```python
from build123d import *

# Parameters (mm, degrees)
F0_W     = 102.9875054955
F0_H     = 41.0375036299
F1_DEPTH = 3
F2_W     = 102.9875054955
F2_H     = 41.0375036299
F3_DEPTH = 2


with BuildPart() as f1:
    # F0 (on Top) → F1 (new body)
    with BuildSketch(Plane.XY):
        with Locations((-51.4937527478, -20.518751815)):
            Rectangle(F0_W, F0_H)
    extrude(amount=F1_DEPTH)

    # F2 (on face) → F3 (join)
    with BuildSketch(Plane.XY.offset(3)):
        with Locations((-51.4937527478, -20.518751815)):
            Rectangle(F2_W, F2_H)
        with BuildLine():
            add(Edge.make_bspline(
                [(-61.8547136732, -13.5894833709), (-60.7502540071, -13.4974450654), (-59.601018949, -13.4974450654)],
                knots=[0, 0, 0, 1, 1, 1], degree=2))
            add(Edge.make_bspline(
                [(-59.601018949, -13.4974450654), (-54.1135459231, -13.4974450654), (-54.1135459231, -17.5371804208)],
                knots=[0, 0, 0, 1, 1, 1], degree=2))
            Line((-54.1135459231, -17.5371804208), (-54.1135459231, -27.0395135845))
            Line((-54.1135459231, -27.0395135845), (-52.650883122, -27.4126418501))
            Line((-52.650883122, -27.4126418501), (-52.650883122, -28.4375008196))
            Line((-52.650883122, -28.4375008196), (-58.02890519, -28.4375008196))
            Line((-58.02890519, -28.4375008196), (-58.3721831944, -27.3181160228))
            add(Edge.make_bspline(
                [(-58.3721831944, -27.3181160228), (-59.5860938184, -28.1439732506), (-60.5636898743, -28.4474509066)],
                knots=[0, 0, 0, 1, 1, 1], degree=2))
            add(Edge.make_bspline(
                [(-60.5636898743, -28.4474509066), (-61.5412859301, -28.7509285627), (-62.5362946383, -28.7509285627)],
                knots=[0, 0, 0, 1, 1, 1], degree=2))
            add(Edge.make_bspline(
                [(-62.5362946383, -28.7509285627), (-67.0635842608, -28.7509285627), (-67.0635842608, -24.3927904206)],
                knots=[0, 0, 0, 1, 1, 1], degree=2))
            add(Edge.make_bspline(
                [(-67.0635842608, -24.3927904206), (-67.0635842608, -22.7460510085), (-66.3944409045, -21.7585048655)],
                knots=[0, 0, 0, 1, 1, 1], degree=2))
            add(Edge.make_bspline(
                [(-66.3944409045, -21.7585048655), (-65.7252975482, -20.7709587226), (-64.4666115323, -20.2983295862)],
                knots=[0, 0, 0, 1, 1, 1], degree=2))
            add(Edge.make_bspline(
                [(-64.4666115323, -20.2983295862), (-63.2079255164, -19.8257004498), (-60.50150183, -19.7610248837)],
                knots=[0, 0, 0, 1, 1, 1], degree=2))
            Line((-60.50150183, -19.7610248837), (-58.6060102408, -19.7162494919))
            Line((-58.6060102408, -19.7162494919), (-58.6060102408, -17.5869308562))
            add(Edge.make_bspline(
                [(-58.6060102408, -17.5869308562), (-58.6060102408, -14.9402076923), (-60.7651791377, -14.9402076923)],
                knots=[0, 0, 0, 1, 1, 1], degree=2))
            add(Edge.make_bspline(
                [(-60.7651791377, -14.9402076923), (-62.073615589, -14.9402076923), (-63.6905047399, -15.7511397895)],
                knots=[0, 0, 0, 1, 1, 1], degree=2))
            Line((-63.6905047399, -15.7511397895), (-64.2775598778, -17.5720057256))
            Line((-64.2775598778, -17.5720057256), (-65.3073938908, -17.5720057256))
            Line((-65.3073938908, -17.5720057256), (-65.3073938908, -14.0397248114))
            add(Edge.make_bspline(
                [(-65.3073938908, -14.0397248114), (-62.9591733393, -13.6815216764), (-61.8547136732, -13.5894833709)],
                knots=[0, 0, 0, 1, 1, 1], degree=2))
        make_face(mode=Mode.SUBTRACT)
        with BuildLine():
            Line((-45.6360717289, -13.8208228956), (-45.4221448567, -15.0994090857))
            Line((-45.4221448567, -15.0994090857), (-44.3624605824, -14.5521542961))
            add(Edge.make_bspline(
                [(-44.3624605824, -14.5521542961), (-42.1883665549, -13.4327694994), (-40.4620264461, -13.4327694994)],
                knots=[0, 0, 0, 1, 1, 1], degree=2))
            add(Edge.make_bspline(
                [(-40.4620264461, -13.4327694994), (-37.850128587, -13.4327694994), (-36.9794959673, -15.3332361321)],
                knots=[0, 0, 0, 1, 1, 1], degree=2))
            add(Edge.make_bspline(
                [(-36.9794959673, -15.3332361321), (-33.7904930574, -13.4327694994), (-31.6014738993, -13.4327694994)],
                knots=[0, 0, 0, 1, 1, 1], degree=2))
            add(Edge.make_bspline(
                [(-31.6014738993, -13.4327694994), (-27.6512893276, -13.4327694994), (-27.6512893276, -17.741157206)],
                knots=[0, 0, 0, 1, 1, 1], degree=2))
            Line((-27.6512893276, -17.741157206), (-27.6512893276, -27.0395135845))
            Line((-27.6512893276, -27.0395135845), (-26.1886265265, -27.4126418501))
            Line((-26.1886265265, -27.4126418501), (-26.1886265265, -28.4375008196))
            Line((-26.1886265265, -28.4375008196), (-33.4472150531, -28.4375008196))
            Line((-33.4472150531, -28.4375008196), (-33.4472150531, -27.4126418501))
            Line((-33.4472150531, -27.4126418501), (-32.1437536453, -27.0395135845))
            Line((-32.1437536453, -27.0395135845), (-32.1437536453, -18.348112518))
            add(Edge.make_bspline(
                [(-32.1437536453, -18.348112518), (-32.1437536453, -17.0396760667), (-32.6487205647, -16.3108321879)],
                knots=[0, 0, 0, 1, 1, 1], degree=2))
            add(Edge.make_bspline(
                [(-32.6487205647, -16.3108321879), (-33.1536874841, -15.5819883091), (-34.1785464536, -15.5819883091)],
                knots=[0, 0, 0, 1, 1, 1], degree=2))
            add(Edge.make_bspline(
                [(-34.1785464536, -15.5819883091), (-35.3327565552, -15.5819883091), (-36.6660682242, -16.233719013)],
                knots=[0, 0, 0, 1, 1, 1], degree=2))
            add(Edge.make_bspline(
                [(-36.6660682242, -16.233719013), (-36.5118418744, -16.8854497169), (-36.5118418744, -17.741157206)],
                knots=[0, 0, 0, 1, 1, 1], degree=2))
            Line((-36.5118418744, -17.741157206), (-36.5118418744, -27.0395135845))
            Line((-36.5118418744, -27.0395135845), (-35.0491790733, -27.4126418501))
            Line((-35.0491790733, -27.4126418501), (-35.0491790733, -28.4375008196))
            Line((-35.0491790733, -28.4375008196), (-42.3127426434, -28.4375008196))
            Line((-42.3127426434, -28.4375008196), (-42.3127426434, -27.4126418501))
            Line((-42.3127426434, -27.4126418501), (-41.0043061921, -27.0395135845))
            Line((-41.0043061921, -27.0395135845), (-41.0043061921, -18.348112518))
            add(Edge.make_bspline(
                [(-41.0043061921, -18.348112518), (-41.0043061921, -17.0396760667), (-41.5092731115, -16.3108321879)],
                knots=[0, 0, 0, 1, 1, 1], degree=2))
            add(Edge.make_bspline(
                [(-41.5092731115, -16.3108321879), (-42.014240031, -15.5819883091), (-43.0415865222, -15.5819883091)],
                knots=[0, 0, 0, 1, 1, 1], degree=2))
            add(Edge.make_bspline(
                [(-43.0415865222, -15.5819883091), (-44.0689330135, -15.5819883091), (-45.3873195519, -16.1839685776)],
                knots=[0, 0, 0, 1, 1, 1], degree=2))
            Line((-45.3873195519, -16.1839685776), (-45.3873195519, -27.0395135845))
            Line((-45.3873195519, -27.0395135845), (-44.0540078829, -27.4126418501))
            Line((-44.0540078829, -27.4126418501), (-44.0540078829, -28.4375008196))
            Line((-44.0540078829, -28.4375008196), (-51.3125964094, -28.4375008196))
            Line((-51.3125964094, -28.4375008196), (-51.3125964094, -27.4126418501))
            Line((-51.3125964094, -27.4126418501), (-49.8847589131, -27.0395135845))
            Line((-49.8847589131, -27.0395135845), (-49.8847589131, -15.2237851742))
            Line((-49.8847589131, -15.2237851742), (-51.3125964094, -14.8506569086))
            Line((-51.3125964094, -14.8506569086), (-51.3125964094, -13.8208228956))
            Line((-51.3125964094, -13.8208228956), (-45.6360717289, -13.8208228956))
        make_face(mode=Mode.SUBTRACT)
        with BuildLine():
            add(Edge.make_bspline(
                [(-74.2475471343, -28.36785021), (-76.4863167278, -28.7509285627), (-78.4116585783, -28.7509285627)],
                knots=[0, 0, 0, 1, 1, 1], degree=2))
            add(Edge.make_bspline(
                [(-78.4116585783, -28.7509285627), (-83.6503794271, -28.7509285627), (-86.5881426382, -25.9673917014)],
                knots=[0, 0, 0, 1, 1, 1], degree=2))
            add(Edge.make_bspline(
                [(-86.5881426382, -25.9673917014), (-89.5259058493, -23.1838548401), (-89.5259058493, -18.2535866908)],
                knots=[0, 0, 0, 1, 1, 1], degree=2))
            add(Edge.make_bspline(
                [(-89.5259058493, -18.2535866908), (-89.5259058493, -12.905414884), (-86.719981292, -10.129340588)],
                knots=[0, 0, 0, 1, 1, 1], degree=2))
            add(Edge.make_bspline(
                [(-86.719981292, -10.129340588), (-83.9140567348, -7.353266292), (-78.4265837089, -7.353266292)],
                knots=[0, 0, 0, 1, 1, 1], degree=2))
            add(Edge.make_bspline(
                [(-78.4265837089, -7.353266292), (-74.8047520109, -7.353266292), (-70.9192430052, -8.3980254357)],
                knots=[0, 0, 0, 1, 1, 1], degree=2))
            Line((-70.9192430052, -8.3980254357), (-70.824717178, -13.4029192381))
            Line((-70.824717178, -13.4029192381), (-72.222704413, -13.4029192381))
            Line((-72.222704413, -13.4029192381), (-72.6605082447, -10.3880428522))
            add(Edge.make_bspline(
                [(-72.6605082447, -10.3880428522), (-74.7102261836, -8.9900556171), (-77.4315750006, -8.9900556171)],
                knots=[0, 0, 0, 1, 1, 1], degree=2))
            add(Edge.make_bspline(
                [(-77.4315750006, -8.9900556171), (-81.038481568, -8.9900556171), (-82.7026336325, -11.2362877759)],
                knots=[0, 0, 0, 1, 1, 1], degree=2))
            add(Edge.make_bspline(
                [(-82.7026336325, -11.2362877759), (-84.3667856971, -13.4825199348), (-84.3667856971, -18.2088112989)],
                knots=[0, 0, 0, 1, 1, 1], degree=2))
            add(Edge.make_bspline(
                [(-84.3667856971, -18.2088112989), (-84.3667856971, -22.5768995281), (-82.6255204576, -24.8629320352)],
                knots=[0, 0, 0, 1, 1, 1], degree=2))
            add(Edge.make_bspline(
                [(-82.6255204576, -24.8629320352), (-80.8842552182, -27.1489645424), (-77.5559510892, -27.1489645424)],
                knots=[0, 0, 0, 1, 1, 1], degree=2))
            add(Edge.make_bspline(
                [(-77.5559510892, -27.1489645424), (-75.7997607191, -27.1489645424), (-74.4863492243, -26.6813104495)],
                knots=[0, 0, 0, 1, 1, 1], degree=2))
            add(Edge.make_bspline(
                [(-74.4863492243, -26.6813104495), (-73.1729377294, -26.2136563567), (-72.4266811982, -25.5768507834)],
                knots=[0, 0, 0, 1, 1, 1], degree=2))
            Line((-72.4266811982, -25.5768507834), (-71.9291768441, -22.1540208271))
            Line((-71.9291768441, -22.1540208271), (-70.5162644784, -22.1540208271))
            Line((-70.5162644784, -22.1540208271), (-70.6058152621, -27.4424921113))
            add(Edge.make_bspline(
                [(-70.6058152621, -27.4424921113), (-72.0087775408, -27.9847718573), (-74.2475471343, -28.36785021)],
                knots=[0, 0, 0, 1, 1, 1], degree=2))
        make_face(mode=Mode.SUBTRACT)
    extrude(amount=F3_DEPTH)


solid = f1.part
```
Here's how the part is built. I have some questions about the finished solid (model axes, mm). A direction names the side the tool comes from. Give positions to 0.01 mm unless a question says otherwise; leave off trailing zeros. Put each result on its own line as item: value. Start each with the question number.
(1) If we mould it in two halves opening along X, with no side actions, what happens to faces 3 (the flat face through (-49.885, -21, 4)), 4 (the flat face through (-52, -20, 5)), 5 (the flat face through (-102.988, -21, 2))? For each: +X half, -X half, draft (parallel to the pull), parting line (faces both ways), or undercut.
(2) Will this pin go through, and if not, where does the flat tip stop? pin 1 Ø7.5 at (x, y) = (-38.5, -23) entering from +Z.
(3) I want a section at A-A on z = 4. State how many separate pieces and enclosed holes the cut face has, then the cut area to 3 significant figures.
(4) For faces 1 (the flat face through (-52, 0, 2)), 2 (the flat face through (-45.387, -22, 4)), which set-ups out of +Z, -Z, +X, -X, +Y, -Y let a thin tool reach every point of the face, with its end or its side?
(5) I need wall thicknesses on line 1 along X through (y, z) = (-12.5, 3.6); line 2 along Y through (x, z) = (-77, 3.95); line 3 along Z through (x, y) = (-87.5, -13.5). Which ranges of each line are inside material? Lowest first, please. Write a range as [from, to].
Answer block:
1. face 3: undercut
1. face 4: draft
1. face 5: -X half
2. pin 1: z = 5
3. separate pieces: 1
3. enclosed holes: 3
3. area: 3,710 mm^2
4. face 1: +Z, -Z, +X, -X, +Y
4. face 2: +Z
5. line 1: [-102.99, -88.4], [-83.42, -72.35], [-70.84, 0]
5. line 2: [-41.04, -28.7], [-27.14, -9], [-7.39, 0]
5. line 3: [0, 3]
